```python
from build123d import *

# Parameters (mm, degrees)
SKETCH1_W           = 50
SKETCH1_H           = 15
SKETCH1_R           = 1.5
BOSS_EXTRUDE1_DEPTH = 3
SKETCH8_W           = 112
SKETCH8_H           = 28
BOSS_EXTRUDE3_DEPTH = 15
BOSS_EXTRUDE4_DEPTH = 3
FILLET3_R           = 1.5
FILLET4_R           = 2
SKETCH11_W          = 110
SKETCH11_H          = 26
CUT_EXTRUDE1_DEPTH  = 14
FILLET6_R           = 2
FILLET7_R           = 2
FILLET8_R           = 2
FILLET9_R           = 2
SKETCH12_W          = 10
SKETCH12_H          = 18
CUT_EXTRUDE2_DEPTH  = 138
SKETCH14_W          = 5
SKETCH14_H          = 3
BOSS_EXTRUDE5_DEPTH = 15
SKETCH15_W          = 5
SKETCH15_H          = 3
BOSS_EXTRUDE6_DEPTH = 15
FILLET12_R          = 5
FILLET13_R          = 5
FILLET14_R          = 5


with BuildPart() as part:
    # Sketch1 → Boss-Extrude1 (new body)
    with BuildSketch(Plane(origin=(0, 0, -9.678822938), x_dir=(1, 0, 0), z_dir=(0, 1, 0))):
        with Locations((-9.059405941, 3.134884125)):
            Rectangle(SKETCH1_W, SKETCH1_H)
        with Locations(Location((-19.059405941, 5.634884125, 0), (0, 0, 270))):
            Circle(SKETCH1_R, mode=Mode.SUBTRACT)
        with Locations(Location((0.940594059, 5.634884125, 0), (0, 0, 270))):
            Circle(SKETCH1_R, mode=Mode.SUBTRACT)
        with Locations(Location((-32.059405941, 4.884884125, 0), (0, 0, 270))):
            Circle(SKETCH1_R, mode=Mode.SUBTRACT)
        with Locations(Location((13.940594059, 4.884884125, 0), (0, 0, 270))):
            Circle(SKETCH1_R, mode=Mode.SUBTRACT)
    extrude(amount=BOSS_EXTRUDE1_DEPTH)

    # Sketch9 → Boss-Extrude4 (add)
    with BuildSketch(Plane.XZ):
        Polygon((-27.059405941, -10.313707063), (8.940594059, -10.313707063), (11.940594059, -5.313707063), (-30.059405941, -5.313707063), align=None)
    extrude(amount=BOSS_EXTRUDE4_DEPTH)

    # Fillet3
    fillet3_edges = [part.edges().sort_by_distance(p)[0] for p in [
        (-27.059405941, -1.5, -10.313707063),
        (8.940594059, -1.5, -10.313707063),
    ]]
    fillet(fillet3_edges, radius=FILLET3_R)


with BuildPart() as body_2:
    # Sketch8 → Boss-Extrude3 (new body)
    with BuildSketch(Plane.XY.offset(-5.313707063)):
        with Locations((-9.059405941, 1.5)):
            Rectangle(SKETCH8_W, SKETCH8_H)
    extrude(amount=BOSS_EXTRUDE3_DEPTH)

    # Fillet4
    fillet4_edges = [body_2.edges().sort_by_distance(p)[0] for p in [
        (-65.059405941, 15.5, 2.186292937),
        (46.940594059, 15.5, 2.186292937),
        (46.940594059, -12.5, 2.186292937),
        (-65.059405941, -12.5, 2.186292937),
    ]]
    fillet(fillet4_edges, radius=FILLET4_R)

    # Sketch11 → Cut-Extrude1 (cut)
    with BuildSketch(Plane.XY.offset(9.686292937)):
        with Locations((-9.059405941, 1.5)):
            Rectangle(SKETCH11_W, SKETCH11_H)
    extrude(amount=-CUT_EXTRUDE1_DEPTH, mode=Mode.SUBTRACT)

    # Fillet6
    fillet6_edges = [body_2.edges().sort_by_distance(p)[0] for p in [
        (-64.059405941, 14.5, 2.686292937),
    ]]
    fillet(fillet6_edges, radius=FILLET6_R)

    # Fillet7
    fillet7_edges = [body_2.edges().sort_by_distance(p)[0] for p in [
        (-64.059405941, -11.5, 2.686292937),
    ]]
    fillet(fillet7_edges, radius=FILLET7_R)

    # Fillet8
    fillet8_edges = [body_2.edges().sort_by_distance(p)[0] for p in [
        (45.940594059, -11.5, 2.686292937),
    ]]
    fillet(fillet8_edges, radius=FILLET8_R)

    # Fillet9
    fillet9_edges = [body_2.edges().sort_by_distance(p)[0] for p in [
        (45.940594059, 14.5, 2.686292937),
    ]]
    fillet(fillet9_edges, radius=FILLET9_R)

    # Sketch12 → Cut-Extrude2 (cut)
    with BuildSketch(Plane.ZY.offset(65.059405941)):
        with Locations((4.686292937, 1.694698027)):
            Rectangle(SKETCH12_W, SKETCH12_H)
    extrude(amount=-CUT_EXTRUDE2_DEPTH, mode=Mode.SUBTRACT)


with BuildPart() as part_1:
    # Body-Move/Copy1: read off the stored shape, not the designer's step
    # Body-Move/Copy1: moved
    add(part.part.moved(Location((0, 12.5, 0))))


    add(body_2.part)  # Boss-Extrude5 merges body 2
    # Sketch14 → Boss-Extrude5 (add)
    with BuildSketch(Plane(origin=(0, 0, -5.313707063), x_dir=(-1, 0, 0), z_dir=(0, 0, -1))):
        with Locations((36.559405941, 14)):
            Rectangle(SKETCH14_W, SKETCH14_H)
    extrude(amount=BOSS_EXTRUDE5_DEPTH)

    # Sketch15 → Boss-Extrude6 (add)
    with BuildSketch(Plane(origin=(0, 0, -5.313707063), x_dir=(-1, 0, 0), z_dir=(0, 0, -1))):
        with Locations((-18.440594059, 14)):
            Rectangle(SKETCH15_W, SKETCH15_H)
    extrude(amount=BOSS_EXTRUDE6_DEPTH)

    # Fillet12
    fillet12_edges = [part_1.edges().sort_by_distance(p)[0] for p in [
        (20.940594059, 14, -5.313707063),
    ]]
    fillet(fillet12_edges, radius=FILLET12_R)

    # Fillet13
    fillet13_edges = [part_1.edges().sort_by_distance(p)[0] for p in [
        (-39.059405941, 14, -5.313707063),
    ]]
    fillet(fillet13_edges, radius=FILLET13_R)

    # Fillet14
    fillet14_edges = [part_1.edges().sort_by_distance(p)[0] for p in [
        (20.940594059, 14, -20.313707063),
        (-39.059405941, 14, -20.313707063),
    ]]
    fillet(fillet14_edges, radius=FILLET14_R)


solid = part_1.part
```
For this review, take the finished solid that the model builds, in its own axes (mm). A direction names the side the tool comes from. Coordinates: 2 decimals unless noted, no trailing zeros. Write each loop counter-clockwise with the first axis right and the second up, starting at its lowest first coordinate (ties: lowest second). Pieces come first, ordered by that corner, then holes.
(1) Add section A-A on y = -1. Give the boundary of the cut face in (x, z), then the cut area to 3 significant figures.
(2) Wall thickness on probe 1 along Y at (x, z) = (-17, 1); probe 2 along X at (y, z) = (1.25, -3); probe 3 along Z at (x, y) = (-52, -10.25): over which ranges is each line inside the solid? List them lowest first.
(3) Add section B-B on x = -55. Give the boundary of the cut face in (y, z).
(4) The part is to be moulded in two halves that separate along Z. For faces 1 (the face through (-63.46, 13.93, 2.59)), 2 (the face through (-30.795, 13.979, -13.757)), 3 (the face through (-28.796, 11.021, -7.42)), say which applies: +Z half, -Z half, draft (parallel to the pull), parting line (faces both ways), or undercut.
(5) Tool access review of faces 4 (the face through (10.64, 11.02, -7.48)), 5 (the face through (-39.059, 14, -13)), 6 (the face through (45.37, 13.9, 2.59)): name each direction out of +Z, -Z, +X, -X, +Y, -Y from which nothing blocks a thin tool from reaching the whole face with its end or side.
(6) Add section C-C on x = -9. Give the boundary of the cut face in (y, z).
(7) For pin 1 Ø2.5 at (x, z) = (0.94, -15.31) entering from -Y; pin 2 Ø14 at (x, y) = (9.5, -1.5) entering from -Z; pin 3 Ø13 at (x, y) = (-21.5, -1) entering from +Z; pin 4 Ø0.8 at (x, y) = (-64.5, 6) entering from +Z, all flat-tipped, find the tip position at first contact; note any pin that passes through.
Answer sheet:
1. outline: (-65.06, -5.31) - (46.94, -5.31) - (46.94, -0.31) - (45.94, -0.31) - (45.94, -4.31) - (-64.06, -4.31) - (-64.06, -0.31) - (-65.06, -0.31) - close
1. area: 120 mm2
2. probe 1: y = -12.5 to -11.5, 14.5 to 15.5
2. probe 2: x = -65.06 to -64.06, 45.94 to 46.94
2. probe 3: z = -5.31 to -4.31
3. outline: (-12.5, -5.31) - (15.5, -5.31) - (15.5, 9.69) - (14.5, 9.69) - (14.5, -4.31) - (-11.5, -4.31) - (-11.5, 9.69) - (-12.5, 9.69) - close
4. face 1: draft
4. face 2: undercut
4. face 3: -Z half
5. face 4: -Z, +X, -Y
5. face 5: -Z, -X, +Y, -Y
5. face 6: +Z
6. outline: (-12.5, -5.31) - (9.5, -5.31) - (9.5, -10.31) - (12.5, -10.31) - (12.5, -20.31) - (15.5, -20.31) - (15.5, 9.69) - (14.5, 9.69) - (14.5, -4.31) - (-11.5, -4.31) - (-11.5, 9.69) - (-12.5, 9.69) - close
7. pin 1: passes through
7. pin 2: stops at z = -5.31
7. pin 3: stops at z = -4.31
7. pin 4: stops at z = -0.31
